Autodesk Inventor part; units mm, degrees
ref_plane "YZ Plane" through (0, 0, 0) normal (1, 0, 0) x (0, 1, 0)
ref_plane "XZ Plane" through (0, 0, 0) normal (0, 1, 0) x (-1, 0, 0)
ref_plane "XY Plane" through (0, 0, 0) normal (0, 0, 1) x (1, 0, 0)
sketch "Sketch2" plane through (124.0011, 71.4979, 0) normal (0, 0, -1) x (-1, 0, 0)
  line L0 (-1.4859, 28.2151) -> (-1.4859, -1.5861)
  line L1 (-1.4859, -1.5861) -> (34.6281, -1.5861)
  line L2 (34.6281, 28.6132) -> (-1.4859, 28.6132)
  line L3 (-1.4859, 28.6132) -> (-1.4859, 28.2151)
  arc A0 (34.6281, -1.5523) -> (34.6281, 28.5794) centre (34.6281, 13.5135) ccw
  line L4 (34.6281, -1.5861) -> (34.6281, -1.5523)
  line L5 (34.6281, 28.5794) -> (34.6281, 28.6132)
  circle A1 centre (34.6281, 13.5135) radius 7.3816
  point P0 (124.0011, -71.4979)
extrude "Extrusion1" add sketch "Sketch2" against normal blind 10
fillet "Fillet1" radius 1.5 3 edges at (107.43, 100.111, 0) (107.43, 69.9118, 0) (125.487, 84.8124, 0)
fillet "Fillet2" radius 1.5 1 edges at (96.7547, 85.0114, 0)
pattern_circular "Circular Pattern1" count 2 over 270 about axis through (125.487, 69.9118, 10) along (0, 1, 0) of "Extrusion1"
properties part number "90joint"
The listing builds one solid part. Answer for the finished solid, in the listing's coordinates (mm). A direction names the side the tool comes from. Round coordinates to 2 decimals unless told otherwise and drop trailing zeros. Order: outer loops, then holes, each group sorted by start corner. A loop starts at its lowest first (then second) coordinate and runs counter-clockwise, first axis right, second up. Notation, with made-up numbers: (78, 56) -> (96, 56) arc R18 ccw to (96, 84) -> close; hole circle Ø11 at (-8.5, 87.25). An arc over 180 degrees is marked (long way). Write each question's results on one line, items separated by ' | '. Start each with the question number.
Q1. Find section D-D (x = 119). Determine the outline of the cut face in (y, z).
Q2. Find section C-C (y = 73). Determine the outline of the cut face in (x, z), then the cut area to 3 significant figures.
Q3. The mould has two halves that part along Y. Classify faces 1 (the cylindrical face through (130.56, 82.18, -32.93)), 2 (the cylindrical face through (130.557, 84.68, -41.176)), 3 (the cylindrical face through (90.973, 77.805, 5.69)), 4 (the cylindrical face through (103.73, 99.66, 0.43)): pulls with the +Y half, pulls with the -Y half, needs draft (parallel to the pull), parting line crosses it, or undercut.
Q4. Find section A-A (z = -30.5). Determine the outline of the cut face in (x, y).
Q5. Each of these flat-tipped pins is pushed along its axis until it touches: pin 1 (13.5 mm diameter, centred on x = 107, y = 88, fed in from -Z); pin 2 (1 mm diameter, centred on y = 83.5, z = -13.5, fed in from -X); pin 3 (12 mm diameter, centred on y = 77.5, z = -2.5, fed in from -X); pin 4 (13.5 mm diameter, centred on x = 89.37, y = 85.01, fed in from +Z). Where does it stop, or does it pass through?
Q6. Which of the six approach directions +Z, -Z, +X, -X, +Y, -Y give full straight-line access (tool end or side, diameter ignored) to faces 5 (the cylindrical face through (103.89, 70.36, 0.43)), 6 (the flat face through (105, 85, 0)), 7 (the flat face through (135.487, 85, -10))?
Q7. Straight lines are drawn through the part: probe 1 along Z at (x, y) = (87, 75.5); probe 2 along X at (y, z) = (72.5, -15.5); probe 3 along Y at (x, z) = (85.5, 4.5). For each, find the intervals that lie inside material, in ascending order. Write a range as from..to.
Worked answers:
1) outline: (69.91, 1.5) arc R1.5 ccw to (71.41, 0) -> (98.61, 0) arc R1.5 ccw to (100.11, 1.5) -> (100.11, 10) -> (69.91, 10) -> close
2) outline: (80.28, 0) -> (123.99, 0) arc R1.5 ccw to (125.49, 1.5) -> (125.49, -35.21) -> (135.49, -35.21) -> (135.49, 10) -> (80.28, 10) -> close | area: 904 mm2
3) face 1: undercut | face 2: parting line crosses it | face 3: undercut | face 4: pulls with the +Y half
4) outline: (125.49, 70.6) -> (135.49, 70.6) -> (135.49, 79.07) -> (125.49, 79.07) -> close; (125.49, 90.95) -> (135.49, 90.95) -> (135.49, 99.42) -> (125.49, 99.42) -> close
5) pin 1: stops at z = 0 | pin 2: stops at x = 125.49 | pin 3: stops at x = 74.45 | pin 4: passes through
6) face 5: -Z, -X, -Y | face 6: -Z, -X, +Y, -Y | face 7: +Z, -Z, +X, +Y, -Y
7) probe 1: z = 0..10 | probe 2: x = 125.49..135.49 | probe 3: y = 70.45..78.73, 91.3..99.57
